from build123d import *

# Parameters (mm, degrees)
F0_W     = 25.4
F0_H     = 25.4
F1_DEPTH = 25.4
F3_DEPTH = 25.4
F2_W     = 1.27
F2_H     = 1.27
F4_DEPTH = 25.4


# Not quite as in the source:
# - the program builds the solid bodies; features that only make, move or delete a surface that nothing else refers to are left out


with BuildPart() as f1:
    # F0 (on Front) → F1 (new body)
    with BuildSketch(Plane.XZ):
        with Locations((-12.7, 12.7)):
            Rectangle(F0_W, F0_H)
    extrude(amount=F1_DEPTH)

    # F2 (on face) → F3 (cut)
    with BuildSketch(Plane.XZ):
        Polygon((-3.9930980909, 15.1806421435), (-5.8980980909, 15.1806421435), (-5.8980980909, 0), (0, 0), (0, 25.4), (-13.5180980909, 25.4), align=None)
        Polygon((-25.4, 0), (-21.1380980909, 0), (-21.1380980909, 15.1806421435), (-23.0430980909, 15.1806421435), (-13.5180980909, 25.4), (-25.4, 25.4), align=None)
    extrude(amount=F3_DEPTH, mode=Mode.SUBTRACT)

    # F2 (on face) → F4 (cut)
    with BuildSketch(Plane.XZ):
        with Locations((-17.9630980909, 11.43)):
            Rectangle(F2_W, F2_H)
        with Locations((-17.9630980909, 8.89)):
            Rectangle(F2_W, F2_H)
        with Locations((-15.4230980909, 11.43)):
            Rectangle(F2_W, F2_H)
        with Locations((-15.4230980909, 8.89)):
            Rectangle(F2_W, F2_H)
        with Locations((-10.9780980909, 8.89)):
            Rectangle(F2_W, F2_H)
        with Locations((-8.4380980909, 8.89)):
            Rectangle(F2_W, F2_H)
        with Locations((-10.9780980909, 11.43)):
            Rectangle(F2_W, F2_H)
        with Locations((-8.4380980909, 11.43)):
            Rectangle(F2_W, F2_H)
    extrude(amount=F4_DEPTH, mode=Mode.SUBTRACT)


solid = f1.part
Build history of the part. All positions in model axes, mm. A direction names the side the tool comes from. Round coordinates to 2 decimals unless told otherwise and drop trailing zeros. Loops run counter-clockwise (first coordinate to the right, second up) from the corner with the lowest first, then second, coordinate; pieces in that order, holes last. Notation, with made-up numbers: (86, -23) -> (125, -23) arc R26 ccw to (125, -9) -> close; hole circle Ø1 at (4, 19). An arc over 180 degrees is marked (long way). Use CSV: the item, a comma, the result in double quotes. Start each with the question number.
Q1. Mould opens along X. For faces 3 (the face through (-8.82, -12.52, 20.36)), 4 (the face through (-15, -13, 8.255)), 5 (the face through (-18, -13, 9.525)), 6 (the face through (-22, -13, 15.181)) say: +X half, -X half, draft (parallel to the pull), parting line (faces both ways), or undercut.
Q2. Saw through at B-B on y = -2.25. Count the separate pieces of the cut face and the enclosed holes in it, and give its area (3 significant figures).
Q3. Which spindle directions (+Z, -Z, +X, -X, +Y, -Y) get a long thin tool onto all of the face, cutting with end or side? Do faces 1 (the face through (-17.328, -13, 11)), 2 (the face through (-14, -25.4, 10)). Say none if no direction does.
Q4. Saw through at A-A on x = -8.25. Give the cut face in (y, z) (3 decimals), and give its area (3 significant figures).
Q5. Saw through at C-C on z = 4.5. Give the cut face in (x, y).
Q6. Drill centre lines: L1, parallel to Z at x = -16, y = -7 (3 decimals); L2, parallel to X at y = -1.5, z = 7.75; L3, parallel to Z at x = -10.75, y = -19.75 (3 decimals). Where is each one in solid material? Low to high.
Q7. Flat gauge pins, fed straight in: pin 1 Ø3 at (x, y) = (-8, -9.5) entering from +Z; pin 2 Ø1.4 at (x, y) = (-11, -9.5) entering from +Z; pin 3 Ø1 at (y, z) = (-11, 9) entering from +X. Where does each tip first touch, or does it go through?
Q8. Saw through at D-D on x = -21.5. Give the cut face in (y, z).
Solutions:
1,face 3,"+X half"
1,face 4,"undercut"
1,face 5,"undercut"
1,face 6,"draft"
2,separate pieces,"1"
2,enclosed holes,"8"
2,area,"316 mm^2"
3,face 1,"+Y, -Y"
3,face 2,"+Z, -Z, +X, -X, -Y"
4,outline,"(-25.4, 0) -> (0, 0) -> (0, 8.255) -> (-25.4, 8.255) -> close; (-25.4, 9.525) -> (0, 9.525) -> (0, 10.795) -> (-25.4, 10.795) -> close; (-25.4, 12.065) -> (0, 12.065) -> (0, 19.748) -> (-25.4, 19.748) -> close"
4,area,"437 mm^2"
5,outline,"(-21.14, -25.4) -> (-5.9, -25.4) -> (-5.9, 0) -> (-21.14, 0) -> close"
6,L1,"z = 0 to 8.255, 9.525 to 10.795, 12.065 to 22.737"
6,L2,"x = -21.14 to -5.9"
6,L3,"z = 0 to 8.255, 9.525 to 10.795, 12.065 to 22.43"
7,pin 1,"stops at z = 21.09"
7,pin 2,"stops at z = 23.45"
7,pin 3,"stops at x = -5.9"
8,outline,"(-25.4, 15.18) -> (0, 15.18) -> (0, 16.84) -> (-25.4, 16.84) -> close"
